The listing builds one solid part. Answer for the finished solid, in the listing's coordinates (mm). Coordinates: 2 decimals unless noted, no trailing zeros. Order: outer loops, then holes, each group sorted by start corner. A loop starts at its lowest first (then second) coordinate and runs counter-clockwise, first axis right, second up. Notation, with made-up numbers: (-18.75, -18) -> (-1.75, -18) arc R34 cw to (-1.75, 13) -> close; hole circle Ø3 at (66, 83). An arc over 180 degrees is marked (long way). One line per question, with ' | ' between items.
from build123d import *

# Parameters (mm, degrees)
SKETCH_1_W          = 30
SKETCH_1_H          = 20
EXTRUDE_1_DEPTH     = 10
FILLET_1_R          = 2
SKETCH_2_R          = 1.7
CUT_EXTRUDE_1_DEPTH = 21.615528128
CUT_EXTRUDE_2_DEPTH = 21.615528128
FILLET_2_R          = 1


with BuildPart() as part:
    # 草图1 → 凸台-拉伸1 (new body)
    with BuildSketch(Plane.XY):
        Rectangle(SKETCH_1_W, SKETCH_1_H)
    extrude(amount=EXTRUDE_1_DEPTH)

    # 圆角1
    fillet_1_edges = [part.edges().sort_by_distance(p)[0] for p in [
        (15, -10, 5),
        (-15, -10, 5),
        (-15, 10, 5),
        (15, 10, 5),
    ]]
    fillet(fillet_1_edges, radius=FILLET_1_R)

    # 草图2 → 切除-拉伸1 (cut, through all)
    with BuildSketch(Plane.XY.offset(10)):
        with Locations((5, 0)):
            Circle(SKETCH_2_R)
        with Locations(Location((-5, 0, 0), (0, 0, 180))):
            Circle(SKETCH_2_R)
    extrude(amount=-CUT_EXTRUDE_1_DEPTH, mode=Mode.SUBTRACT)

    # 草图3 → 切除-拉伸2 (cut, through all)
    with BuildSketch(Plane.XY.offset(10)):
        Polygon((-13, 2), (-13, 8), (-2, 8), (-2, 4), (-9, 4), (-9, 2), align=None)
        Polygon((9, 2), (13, 2), (13, 8), (2, 8), (2, 4), (9, 4), align=None)
        Polygon((13, -2), (13, -8), (2, -8), (2, -4), (9, -4), (9, -2), align=None)
        Polygon((-9, -2), (-13, -2), (-13, -8), (-2, -8), (-2, -4), (-9, -4), align=None)
    extrude(amount=-CUT_EXTRUDE_2_DEPTH, mode=Mode.SUBTRACT)

    # 圆角2
    fillet_2_edges = [part.edges().sort_by_distance(p)[0] for p in [
        (-2, -4, 5),
        (2, 8, 5),
        (13, 8, 5),
        (13, 2, 5),
        (2, 4, 5),
        (9, 2, 5),
        (9, 4, 5),
        (13, -2, 5),
        (2, -8, 5),
        (2, -4, 5),
        (9, -2, 5),
        (9, -4, 5),
        (13, -8, 5),
        (-2, -8, 5),
        (-13, -8, 5),
        (-13, -2, 5),
        (-9, -2, 5),
        (-9, -4, 5),
        (-2, 8, 5),
        (-2, 4, 5),
        (-9, 4, 5),
        (-9, 2, 5),
        (-13, 2, 5),
        (-13, 8, 5),
    ]]
    fillet(fillet_2_edges, radius=FILLET_2_R - 0.0001)  # a hair under: the kernel refuses the full size


solid = part.part
Item 1: Section C-C, the plane z = 8.5 is taken. Count the separate pieces of the cut face and the enclosed holes in it, plus the area to 3 significant figures.
Computed values:
separate pieces: 1 | enclosed holes: 6 | area: 374 mm^2
Item 2: Determine the mould class of faces 1 (the face through (-14.43, -9.4, 5.07)), 2 (the face through (-14.43, 9.4, 5.07)), 3 (the face through (11, 2, 5)) for opening direction Y: pulls with the +Y half, pulls with the -Y half, needs draft (parallel to the pull), parting line crosses it, or undercut.
Computed values:
face 1: pulls with the -Y half | face 2: pulls with the +Y half | face 3: undercut
Item 3: This flat-tipped pin is pushed along its axis until it touches: pin 1 Ø1.5 at (x, y) = (-4.5, 0) entering from +Z. Where does it stop, or does it pass through?
Computed values:
pin 1: passes through
Item 4: Section A-A, the plane y = 0 is taken. Give the vertices of the cut face in (x, z).
Computed values:
outline: (-15, 0) -> (-6.7, 0) -> (-6.7, 10) -> (-15, 10) -> close; (-3.3, 0) -> (3.3, 0) -> (3.3, 10) -> (-3.3, 10) -> close; (6.7, 0) -> (15, 0) -> (15, 10) -> (6.7, 10) -> close
Item 5: Section B-B, the plane x = 5 is taken. Give the vertices of the cut face in (y, z).
Computed values:
outline: (-10, 0) -> (-8, 0) -> (-8, 10) -> (-10, 10) -> close; (-4, 0) -> (-1.7, 0) -> (-1.7, 10) -> (-4, 10) -> close; (1.7, 0) -> (4, 0) -> (4, 10) -> (1.7, 10) -> close; (8, 0) -> (10, 0) -> (10, 10) -> (8, 10) -> close
Item 6: Find the intervals of material crossed by L1, parallel to X at y = -3, z = 3; L2, parallel to Y at x = 5, z = 4.25; L3, parallel to X at y = 7, z = 2.5, in increasing order.
Computed values:
L1: x = -15 to -13, -9 to 9, 13 to 15 | L2: y = -10 to -8, -4 to -1.7, 1.7 to 4, 8 to 10 | L3: x = -15 to -13, -2 to 2, 13 to 15
Item 7: Section D-D, the plane y = -6.5 is taken. Give the vertices of the cut face in (x, z), plus the area to 3 significant figures.
Computed values:
outline: (-15, 0) -> (-13, 0) -> (-13, 10) -> (-15, 10) -> close; (-2, 0) -> (2, 0) -> (2, 10) -> (-2, 10) -> close; (13, 0) -> (15, 0) -> (15, 10) -> (13, 10) -> close | area: 80.0 mm^2
